Geometry: see drawing. Coordinates: mm, zero at the bounding-box minimum. Coordinates: 2 decimals unless noted, no trailing zeros. Loops run counter-clockwise (first coordinate to the right, second up) from the corner with the lowest first, then second, coordinate; pieces in that order, holes last. Notation, with made-up numbers: (53.5, 31.25) - (65.5, 31.25) arc R20 ccw to (65.5, 62.25) - close; hole circle Ø3 at (22, 56). An arc over 180 degrees is marked (long way). Use one line per item in the form item = value.
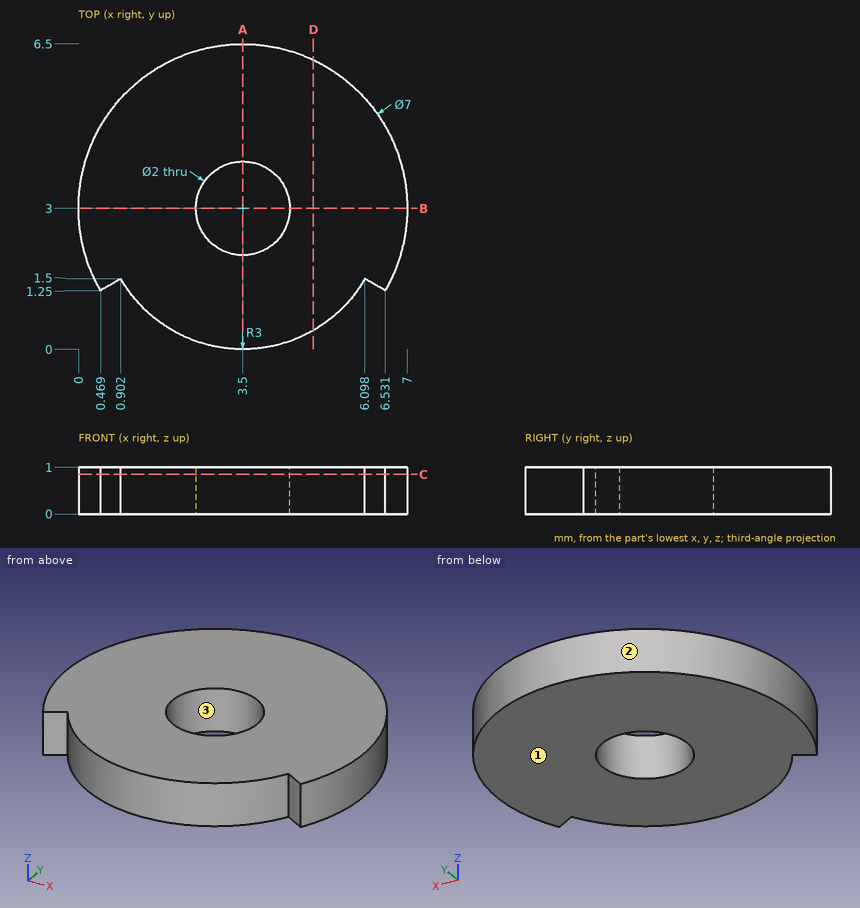
Q1. Ray query, line 1 along X through (y, z) = (3, 0.7); line 2 along Y through (x, z) = (3.5, 0.2); line 3 along Y through (x, z) = (2.75, 0.8) (1 decimal). Return the intervals inside material, ascending. Write a range as [from, to].
Check values:
line_1 = [0, 2.5], [4.5, 7]
line_2 = [0, 2], [4, 6.5]
line_3 = [0.1, 2.3], [3.7, 6.4]
Q2. Cut plane A-A, the plane x = 3.5. Return loops of the section in (y, z).
Check values:
outline = (0, 0) - (2, 0) - (2, 1) - (0, 1) - close; (4, 0) - (6.5, 0) - (6.5, 1) - (4, 1) - close
Q3. Cut plane C-C, the plane z = 0.85. Return loops of the section in (x, y), then the cut area to 3 significant figures.
Check values:
outline = (0.47, 1.25) - (0.9, 1.5) arc R3 ccw to (6.1, 1.5) - (6.53, 1.25) arc R3.5 ccw (long way) to start; hole circle Ø2 at (3.5, 3)
area = 31.9 mm²
Q4. Cut plane D-D, the plane x = 5. Return loops of the section in (y, z).
Check values:
outline = (0.4, 0) - (6.16, 0) - (6.16, 1) - (0.4, 1) - close
Q5. Cut plane B-B, the plane y = 3. Return loops of the section in (x, z), then the cut area to 3 significant figures.
Check values:
outline = (0, 0) - (2.5, 0) - (2.5, 1) - (0, 1) - close; (4.5, 0) - (7, 0) - (7, 1) - (4.5, 1) - close
area = 5.00 mm²
Q6. Pull-direction query (X, two-part tool) for the marked faces 1, 2 and 3; classes: pulls with the +X half, pulls with the -X half, needs draft (parallel to the pull), parting line crosses it, or undercut.
Check values:
face_1 = needs draft
face_2 = parting line crosses it
face_3 = undercut
